Job drawing, mm, ordinate dimensions from the low corner. One solid piece. A direction names the side the tool comes from. Give positions to 0.01 mm unless a question says otherwise; leave off trailing zeros. Write each loop counter-clockwise with the first axis right and the second up, starting at its lowest first coordinate (ties: lowest second). Pieces come first, ordered by that corner, then holes. Notation, with made-up numbers: (40.25, 74.25) -> (69.25, 74.25) arc R30 ccw to (69.25, 110.25) -> close; hole circle Ø4 at (84.25, -36.75). An arc over 180 degrees is marked (long way). Put each result on its own line as item: value. Start each with the question number.
Item 1: Two-plate mould, pull along Z, no slides. Class the marked faces 4 and 5: pulls with the +Z half, pulls with the -Z half, needs draft (parallel to the pull), parting line crosses it, or undercut.
Item 2: Slice it at A-A, the plane y = 1.35. List the corners of the cut face in (x, z), plus the area to 3 significant figures.
Item 3: Slice it at B-B, the plane x = 4.25. List the corners of the cut face in (y, z), plus the area to 3 significant figures.
Item 4: Drill centre lines: line 1 along X through (y, z) = (1.35, 6); line 2 along Z through (x, y) = (16.5, 1.6); line 3 along Z through (x, y) = (18.5, 1.8). Where is each one in solid material? Low to high.
Item 5: Slice it at D-D, the plane x = 16. List the corners of the cut face in (y, z).
Item 6: Tool access for the marked faces 1, 2 and 3: list every direction of +Z, -Z, +X, -X, +Y, -Y with a clear straight run to the whole face (end or side of a thin tool).
Item 7: Slice it at C-C, the plane z = 5. List the corners of the cut face in (x, y), plus the area to 3 significant figures.
Item 8: Flat gauge pins, fed straight in: pin 1 Ø0.9 at (y, z) = (1.5, 5.5) entering from +X; pin 2 Ø0.9 at (x, y) = (12, 1.5) entering from -Z; pin 3 Ø0.7 at (y, z) = (1.5, 4) entering from -X. Where does each tip first touch, or does it go through?
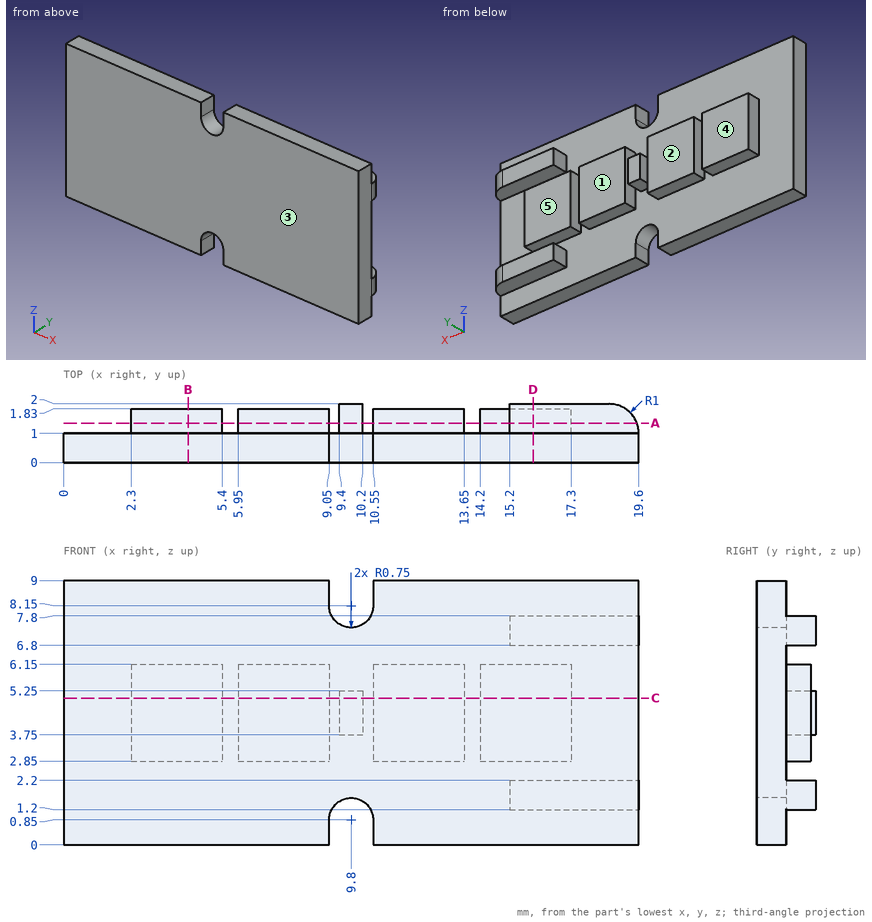
Values follow:
1. face 4: needs draft
1. face 5: undercut
2. outline: (2.3, 2.85) -> (5.4, 2.85) -> (5.4, 6.15) -> (2.3, 6.15) -> close; (5.95, 2.85) -> (9.05, 2.85) -> (9.05, 6.15) -> (5.95, 6.15) -> close; (9.4, 3.75) -> (10.2, 3.75) -> (10.2, 5.25) -> (9.4, 5.25) -> close; (10.55, 2.85) -> (13.65, 2.85) -> (13.65, 6.15) -> (10.55, 6.15) -> close; (14.2, 2.85) -> (17.3, 2.85) -> (17.3, 6.15) -> (14.2, 6.15) -> close; (15.2, 1.2) -> (19.54, 1.2) -> (19.54, 2.2) -> (15.2, 2.2) -> close; (15.2, 6.8) -> (19.54, 6.8) -> (19.54, 7.8) -> (15.2, 7.8) -> close
2. area: 50.8 mm2
3. outline: (0, 0) -> (1, 0) -> (1, 2.85) -> (1.83, 2.85) -> (1.83, 6.15) -> (1, 6.15) -> (1, 9) -> (0, 9) -> close
3. area: 11.7 mm2
4. line 1: 2.3 to 5.4, 5.95 to 9.05, 10.55 to 13.65, 14.2 to 17.3
4. line 2: 1.2 to 2.2, 2.85 to 6.15, 6.8 to 7.8
4. line 3: 1.2 to 2.2, 6.8 to 7.8
5. outline: (0, 0) -> (1, 0) -> (1, 1.2) -> (2, 1.2) -> (2, 2.2) -> (1, 2.2) -> (1, 2.85) -> (1.83, 2.85) -> (1.83, 6.15) -> (1, 6.15) -> (1, 6.8) -> (2, 6.8) -> (2, 7.8) -> (1, 7.8) -> (1, 9) -> (0, 9) -> close
6. face 1: +Z, -Z, +X, +Y
6. face 2: +Z, -Z, -X, +Y
6. face 3: +Z, -Z, +X, -X, -Y
7. outline: (0, 0) -> (19.6, 0) -> (19.6, 1) -> (17.3, 1) -> (17.3, 1.83) -> (14.2, 1.83) -> (14.2, 1) -> (13.65, 1) -> (13.65, 1.83) -> (10.55, 1.83) -> (10.55, 1) -> (10.2, 1) -> (10.2, 2) -> (9.4, 2) -> (9.4, 1) -> (9.05, 1) -> (9.05, 1.83) -> (5.95, 1.83) -> (5.95, 1) -> (5.4, 1) -> (5.4, 1.83) -> (2.3, 1.83) -> (2.3, 1) -> (0, 1) -> close
7. area: 30.7 mm2
8. pin 1: x = 17.3
8. pin 2: z = 2.85
8. pin 3: x = 2.3
